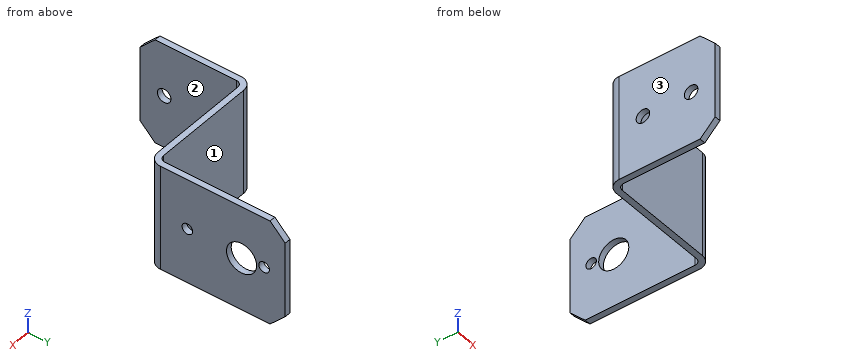
```python
from build123d import *

# Parameters (mm, degrees)
BASE_FLANGE1_DEPTH = 35
SKETCH3_R          = 5
SKETCH3_R_2        = 1.75
CUT_EXTRUDE1_DEPTH = 10
CHAMFER1_SIZE      = 5
SKETCH4_R          = 2.25
CUT_EXTRUDE2_DEPTH = 10


# Sheet-metal steps are written as plain solids
with BuildPart() as part:
    # Sketch1 → Base-Flange1 (new body)
    with BuildSketch(Plane.XY):
        with BuildLine():
            Line((-40, -34), (-40, -2))
            ThreePointArc((-40, -2), (-39.414213562, -0.585786438), (-38, 0))
            Line((-38, 0), (-4, 0))
            ThreePointArc((-4, 0), (-1.171572875, 1.171572875), (0, 4))
            Line((0, 4), (0, 45.5))
            Line((0, 45.5), (-2, 45.5))
            Line((-2, 45.5), (-2, 4))
            ThreePointArc((-2, 4), (-2.585786438, 2.585786438), (-4, 2))
            Line((-4, 2), (-38, 2))
            ThreePointArc((-38, 2), (-40.828427125, 0.828427125), (-42, -2))
            Line((-42, -2), (-42, -34))
            Line((-42, -34), (-40, -34))
        make_face()
    extrude(amount=BASE_FLANGE1_DEPTH)

    # Sketch3 → Cut-Extrude1 (cut)
    with BuildSketch(Plane(origin=(0, 0, 0), x_dir=(0, 0, -1), z_dir=(1, 0, 0))):
        with Locations((-17.5, 31)):
            Circle(SKETCH3_R)
        with Locations((-18.25, 13)):
            Circle(SKETCH3_R_2)
        with Locations((-18.25, 38.5)):
            Circle(SKETCH3_R_2)
    extrude(amount=-CUT_EXTRUDE1_DEPTH, mode=Mode.SUBTRACT)

    # Chamfer1
    chamfer1_edges = [part.edges().sort_by_distance(p)[0] for p in [
        (-1, 45.5, 0),
        (-41, -34, 0),
        (-1, 45.5, 35),
        (-41, -34, 35),
    ]]
    chamfer(chamfer1_edges, length=CHAMFER1_SIZE)

    # Sketch4 → Cut-Extrude2 (cut)
    with BuildSketch(Plane(origin=(-40, 0, 0), x_dir=(0, 0, -1), z_dir=(1, 0, 0))):
        with Locations(Location((-17.5, -26, 0), (0, 0, 90))):
            Circle(SKETCH4_R)
        with Locations(Location((-17.5, -10, 0), (0, 0, 90))):
            Circle(SKETCH4_R)
    extrude(amount=-CUT_EXTRUDE2_DEPTH, mode=Mode.SUBTRACT)


solid = part.part
```
Source: CAD feature listing. Evaluate the final solid. Frame: model axes, mm. Face numbers are marked on the shaded views. A direction names the side the tool comes from. Coordinates: 2 decimals unless noted, no trailing zeros. Loops run counter-clockwise (first coordinate to the right, second up) from the corner with the lowest first, then second, coordinate; pieces in that order, holes last. Notation, with made-up numbers: M -39.5,22 L 6.5,22 A13 cw 6.5,47 Z; hole C 43,8.5 d10. An arc over 180 degrees is marked long. Put each result on its own line as item: value. Start each with the question number.
1) Contact query for flat-ended pins moving along their axis: pin 1 Ø17.5 at (y, z) = (22.5, 17) entering from -X; pin 2 Ø1.5 at (x, z) = (-35, 16) entering from -Y; pin 3 Ø9.5 at (y, z) = (-22, 25.5) entering from +X. Output: stop coordinate, or through.
2) Cut plane B-B on z = 17.5. Give the number of separate pieces and of enclosed holes in the cut face, then the cut area to 3 significant figures.
3) Cut plane D-D on z = 28.5. Return the cut outline in (x, y), then the cut area to 3 significant figures.
4) Reachability of the marked faces 1, 2 and 3 from +Z, -Z, +X, -X, +Y, -Y: full face, straight path, thin tool, end or side. Return the list, or none.
5) Cut plane C-C on y = 38.5. Return the cut outline in (x, z), then the cut area to 3 significant figures.
6) Cut plane A-A on y = -26. Return the cut outline in (x, z).
7) Ray query, L1, parallel to Y at x = -0.4, z = 18.25; L2, parallel to Z at x = -40.75, y = -26; L3, parallel to Y at x = -41, z = 17. Return the intervals inside material, ascending. Write a range as from..to.
The answers:
1. pin 1: stops at x = -2
1. pin 2: stops at y = 0
1. pin 3: stops at x = -40
2. separate pieces: 6
2. enclosed holes: 0
2. area: 183 mm²
3. outline: M -42,-34 L -40,-34 L -40,-2 A2 cw -38,0 L -4,0 A4 ccw 0,4 L 0,45.5 L -2,45.5 L -2,4 A2 cw -4,2 L -38,2 A4 ccw -42,-2 Z
3. area: 234 mm²
4. face 1: +Z, -Z, -X, +Y
4. face 2: +Z, -Z, +X, -Y
4. face 3: +Z, -Z, -X, +Y, -Y
5. outline: M -2,0 L 0,0 L 0,16.5 L -2,16.5 Z; M -2,20 L 0,20 L 0,35 L -2,35 Z
5. area: 63.0 mm²
6. outline: M -42,0 L -40,0 L -40,15.25 L -42,15.25 Z; M -42,19.75 L -40,19.75 L -40,35 L -42,35 Z
7. L1: y = 2.26..11.25, 14.75..26.06, 35.94..36.75, 40.25..45.5
7. L2: z = 0..15.25, 19.75..35
7. L3: y = -34..-28.19, -23.81..-12.19, -7.81..0.65
